```python
from build123d import *

# Parameters (mm, degrees)
SKETCH_1_R      = 3.4
EXTRUDE_1_DEPTH = 10


with BuildPart() as part:
    # 草图1 → 凸台-拉伸1 (new body)
    with BuildSketch(Plane.XY):
        with BuildLine():
            Line((-5.190537873, 20), (-27.590537873, 20))
            ThreePointArc((-27.590537873, 20), (-29.358304826, 19.267766953), (-30.090537873, 17.5))
            Line((-30.090537873, 17.5), (-30.090537873, 5.1))
            Line((-30.090537873, 5.1), (-29.090537873, 5.1))
            Line((-29.090537873, 5.1), (-29.090537873, 4.1))
            Line((-29.090537873, 4.1), (-25.890537873, 4.1))
            ThreePointArc((-25.890537873, 4.1), (-25.678405839, 4.187867966), (-25.590537873, 4.4))
            Line((-25.590537873, 4.4), (-25.590537873, 6.7))
            ThreePointArc((-25.590537873, 6.7), (-25.678405839, 6.912132034), (-25.890537873, 7))
            Line((-25.890537873, 7), (-27.290537873, 7))
            ThreePointArc((-27.290537873, 7), (-27.502669908, 7.087867966), (-27.590537873, 7.3))
            Line((-27.590537873, 7.3), (-27.590537873, 9.95))
            ThreePointArc((-27.590537873, 9.95), (-27.502669908, 10.162132034), (-27.290537873, 10.25))
            Line((-27.290537873, 10.25), (-22.856071779, 10.25))
            Line((-22.856071779, 10.25), (-17.840537873, 5.234466094))
            Line((-17.840537873, 5.234466094), (-17.840537873, 0))
            Line((-17.840537873, 0), (-17.840537873, -5.234466094))
            Line((-17.840537873, -5.234466094), (-22.856071779, -10.25))
            Line((-22.856071779, -10.25), (-27.290537873, -10.25))
            ThreePointArc((-27.290537873, -10.25), (-27.502669908, -10.162132034), (-27.590537873, -9.95))
            Line((-27.590537873, -9.95), (-27.590537873, -7.3))
            ThreePointArc((-27.590537873, -7.3), (-27.502669908, -7.087867966), (-27.290537873, -7))
            Line((-27.290537873, -7), (-25.890537873, -7))
            ThreePointArc((-25.890537873, -7), (-25.678405839, -6.912132034), (-25.590537873, -6.7))
            Line((-25.590537873, -6.7), (-25.590537873, -4.4))
            ThreePointArc((-25.590537873, -4.4), (-25.678405839, -4.187867966), (-25.890537873, -4.1))
            Line((-25.890537873, -4.1), (-29.090537873, -4.1))
            Line((-29.090537873, -4.1), (-29.090537873, -5.1))
            Line((-29.090537873, -5.1), (-30.090537873, -5.1))
            Line((-30.090537873, -5.1), (-30.090537873, -17.5))
            ThreePointArc((-30.090537873, -17.5), (-29.358304826, -19.267766953), (-27.590537873, -20))
            Line((-27.590537873, -20), (-5.190537873, -20))
            Line((-5.190537873, -20), (-5.190537873, -19))
            Line((-5.190537873, -19), (-4.190537873, -19))
            Line((-4.190537873, -19), (-4.190537873, -15.8))
            ThreePointArc((-4.190537873, -15.8), (-4.278405839, -15.587867966), (-4.490537873, -15.5))
            Line((-4.490537873, -15.5), (-6.790537873, -15.5))
            ThreePointArc((-6.790537873, -15.5), (-7.002669908, -15.587867966), (-7.090537873, -15.8))
            Line((-7.090537873, -15.8), (-7.090537873, -17.2))
            ThreePointArc((-7.090537873, -17.2), (-7.178405839, -17.412132034), (-7.390537873, -17.5))
            Line((-7.390537873, -17.5), (-10.040537873, -17.5))
            ThreePointArc((-10.040537873, -17.5), (-10.252669908, -17.412132034), (-10.340537873, -17.2))
            Line((-10.340537873, -17.2), (-10.340537873, -12.765533906))
            Line((-10.340537873, -12.765533906), (-5.325003967, -7.75))
            Line((-5.325003967, -7.75), (-0.090537873, -7.75))
            Line((-0.090537873, -7.75), (5.143928221, -7.75))
            Line((5.143928221, -7.75), (10.159462127, -12.765533906))
            Line((10.159462127, -12.765533906), (10.159462127, -17.2))
            ThreePointArc((10.159462127, -17.2), (10.071594161, -17.412132034), (9.859462127, -17.5))
            Line((9.859462127, -17.5), (7.209462127, -17.5))
            ThreePointArc((7.209462127, -17.5), (6.997330092, -17.412132034), (6.909462127, -17.2))
            Line((6.909462127, -17.2), (6.909462127, -15.8))
            ThreePointArc((6.909462127, -15.8), (6.821594161, -15.587867966), (6.609462127, -15.5))
            Line((6.609462127, -15.5), (4.309462127, -15.5))
            ThreePointArc((4.309462127, -15.5), (4.097330092, -15.587867966), (4.009462127, -15.8))
            Line((4.009462127, -15.8), (4.009462127, -19))
            Line((4.009462127, -19), (5.009462127, -19))
            Line((5.009462127, -19), (5.009462127, -20))
            Line((5.009462127, -20), (27.409462127, -20))
            ThreePointArc((27.409462127, -20), (29.17722908, -19.267766953), (29.909462127, -17.5))
            Line((29.909462127, -17.5), (29.909462127, -5.1))
            Line((29.909462127, -5.1), (28.909462127, -5.1))
            Line((28.909462127, -5.1), (28.909462127, -4.1))
            Line((28.909462127, -4.1), (25.709462127, -4.1))
            ThreePointArc((25.709462127, -4.1), (25.497330092, -4.187867966), (25.409462127, -4.4))
            Line((25.409462127, -4.4), (25.409462127, -6.7))
            ThreePointArc((25.409462127, -6.7), (25.497330092, -6.912132034), (25.709462127, -7))
            Line((25.709462127, -7), (27.109462127, -7))
            ThreePointArc((27.109462127, -7), (27.321594161, -7.087867966), (27.409462127, -7.3))
            Line((27.409462127, -7.3), (27.409462127, -9.95))
            ThreePointArc((27.409462127, -9.95), (27.321594161, -10.162132034), (27.109462127, -10.25))
            Line((27.109462127, -10.25), (22.674996033, -10.25))
            Line((22.674996033, -10.25), (17.659462127, -5.234466094))
            Line((17.659462127, -5.234466094), (17.659462127, 0))
            Line((17.659462127, 0), (17.659462127, 5.234466094))
            Line((17.659462127, 5.234466094), (22.674996033, 10.25))
            Line((22.674996033, 10.25), (27.109462127, 10.25))
            ThreePointArc((27.109462127, 10.25), (27.321594161, 10.162132034), (27.409462127, 9.95))
            Line((27.409462127, 9.95), (27.409462127, 7.3))
            ThreePointArc((27.409462127, 7.3), (27.321594161, 7.087867966), (27.109462127, 7))
            Line((27.109462127, 7), (25.709462127, 7))
            ThreePointArc((25.709462127, 7), (25.497330092, 6.912132034), (25.409462127, 6.7))
            Line((25.409462127, 6.7), (25.409462127, 4.4))
            ThreePointArc((25.409462127, 4.4), (25.497330092, 4.187867966), (25.709462127, 4.1))
            Line((25.709462127, 4.1), (28.909462127, 4.1))
            Line((28.909462127, 4.1), (28.909462127, 5.1))
            Line((28.909462127, 5.1), (29.909462127, 5.1))
            Line((29.909462127, 5.1), (29.909462127, 17.5))
            ThreePointArc((29.909462127, 17.5), (29.17722908, 19.267766953), (27.409462127, 20))
            Line((27.409462127, 20), (5.009462127, 20))
            Line((5.009462127, 20), (5.009462127, 19))
            Line((5.009462127, 19), (4.009462127, 19))
            Line((4.009462127, 19), (4.009462127, 15.8))
            ThreePointArc((4.009462127, 15.8), (4.097330092, 15.587867966), (4.309462127, 15.5))
            Line((4.309462127, 15.5), (6.609462127, 15.5))
            ThreePointArc((6.609462127, 15.5), (6.821594161, 15.587867966), (6.909462127, 15.8))
            Line((6.909462127, 15.8), (6.909462127, 17.2))
            ThreePointArc((6.909462127, 17.2), (6.997330092, 17.412132034), (7.209462127, 17.5))
            Line((7.209462127, 17.5), (9.859462127, 17.5))
            ThreePointArc((9.859462127, 17.5), (10.071594161, 17.412132034), (10.159462127, 17.2))
            Line((10.159462127, 17.2), (10.159462127, 12.765533906))
            Line((10.159462127, 12.765533906), (5.143928221, 7.75))
            Line((5.143928221, 7.75), (-0.090537873, 7.75))
            Line((-0.090537873, 7.75), (-5.325003967, 7.75))
            Line((-5.325003967, 7.75), (-10.340537873, 12.765533906))
            Line((-10.340537873, 12.765533906), (-10.340537873, 17.2))
            ThreePointArc((-10.340537873, 17.2), (-10.252669908, 17.412132034), (-10.040537873, 17.5))
            Line((-10.040537873, 17.5), (-7.390537873, 17.5))
            ThreePointArc((-7.390537873, 17.5), (-7.178405839, 17.412132034), (-7.090537873, 17.2))
            Line((-7.090537873, 17.2), (-7.090537873, 15.8))
            ThreePointArc((-7.090537873, 15.8), (-7.002669908, 15.587867966), (-6.790537873, 15.5))
            Line((-6.790537873, 15.5), (-4.490537873, 15.5))
            ThreePointArc((-4.490537873, 15.5), (-4.278405839, 15.587867966), (-4.190537873, 15.8))
            Line((-4.190537873, 15.8), (-4.190537873, 19))
            Line((-4.190537873, 19), (-5.190537873, 19))
            Line((-5.190537873, 19), (-5.190537873, 20))
        make_face()
        with Locations((-0.090537873, 0)):
            Circle(SKETCH_1_R, mode=Mode.SUBTRACT)
        Polygon((-12.840537873, 17.5), (-27.590537873, 17.5), (-27.590537873, 12.75), (-21.820537873, 12.75), (-18.550537873, 9.48), (-12.840537873, 9.48), (-12.840537873, 10.25), (-12.840537873, 12.75), align=None, mode=Mode.SUBTRACT)
        Polygon((-15.340537873, 6.98), (-15.340537873, 0), (-15.340537873, -6.98), (-10.340537873, -6.98), (-10.340537873, -4.48), (-5.990537873, -4.48), (-5.990537873, 0), (-5.990537873, 4.48), (-10.340537873, 4.48), (-10.340537873, 6.98), align=None, mode=Mode.SUBTRACT)
        Polygon((12.659462127, 17.5), (27.409462127, 17.5), (27.409462127, 12.75), (21.639462127, 12.75), (18.369462127, 9.48), (12.659462127, 9.48), (12.659462127, 10.25), (12.659462127, 12.75), align=None, mode=Mode.SUBTRACT)
        Polygon((15.159462127, 6.98), (15.159462127, 0), (15.159462127, -6.98), (10.159462127, -6.98), (10.159462127, -4.48), (5.809462127, -4.48), (5.809462127, 0), (5.809462127, 4.48), (10.159462127, 4.48), (10.159462127, 6.98), align=None, mode=Mode.SUBTRACT)
        Polygon((-12.840537873, -17.5), (-27.590537873, -17.5), (-27.590537873, -12.75), (-21.820537873, -12.75), (-18.550537873, -9.48), (-12.840537873, -9.48), (-12.840537873, -10.25), (-12.840537873, -12.75), align=None, mode=Mode.SUBTRACT)
        Polygon((12.659462127, -17.5), (27.409462127, -17.5), (27.409462127, -12.75), (21.639462127, -12.75), (18.369462127, -9.48), (12.659462127, -9.48), (12.659462127, -10.25), (12.659462127, -12.75), align=None, mode=Mode.SUBTRACT)
    extrude(amount=EXTRUDE_1_DEPTH)


solid = part.part
```
Geometry: final body of the model. Coordinates: model frame, mm. A direction names the side the tool comes from. Coordinates: 2 decimals unless noted, no trailing zeros. Order: outer loops, then holes, each group sorted by start corner. A loop starts at its lowest first (then second) coordinate and runs counter-clockwise, first axis right, second up. Notation, with made-up numbers: (13.25, 50.5) -> (43.25, 50.5) arc R4 ccw to (43.25, 56.5) -> close; hole circle Ø11 at (11.25, -23.75). An arc over 180 degrees is marked (long way). Answer in a Markdown table with one row per item.
Item 1: Section A-A on y = 0. Output: boundary loops of the cut face in (x, z), plus the area to 3 significant figures.
Return value:
| item | result |
|---|---|
| outline | (-17.84, 0) -> (-15.34, 0) -> (-15.34, 10) -> (-17.84, 10) -> close; (-5.99, 0) -> (-3.49, 0) -> (-3.49, 10) -> (-5.99, 10) -> close; (3.31, 0) -> (5.81, 0) -> (5.81, 10) -> (3.31, 10) -> close; (15.16, 0) -> (17.66, 0) -> (17.66, 10) -> (15.16, 10) -> close |
| area | 100 mm² |
Item 2: Ray query, L1, parallel to X at y = -14, z = 0.75; L2, parallel to Y at x = 4.5, z = 0.5; L3, parallel to Y at x = -23.5, z = 3.5. Return the intervals inside material, ascending.
Return value:
| item | result |
|---|---|
| L1 | x = -30.09 to -27.59, -12.84 to -10.34, 10.16 to 12.66, 27.41 to 29.91 |
| L2 | y = -19 to -15.5, -7.75 to 7.75, 15.5 to 19 |
| L3 | y = -20 to -17.5, -12.75 to -10.25, 10.25 to 12.75, 17.5 to 20 |
Item 3: Section C-C on x = -11. Output: boundary loops of the cut face in (y, z), plus the area to 3 significant figures.
Return value:
| item | result |
|---|---|
| outline | (-20, 0) -> (-6.98, 0) -> (-6.98, 10) -> (-20, 10) -> close; (6.98, 0) -> (20, 0) -> (20, 10) -> (6.98, 10) -> close |
| area | 260 mm² |
Item 4: Access query for faces 1 (the flat face through (2, -3, 0)), 2 (the flat face through (-16, -9.48, 5)). Directions: +Z, -Z, +X, -X, +Y, -Y. A direction counts if a zero-diameter tool reaches every point of the face in a straight line with its end or side. Return the directions, or none.
Return value:
| item | result |
|---|---|
| face 1 | -Z, +X, -X, +Y, -Y |
| face 2 | +Z, -Z |
Item 5: Contact query for flat-ended pins moving along their axis: P1, Ø3, axis at y = -1.5, z = 5, coming from the +X side; P2, Ø2, axis at x = 22.5, y = 7, coming from the -Z side; P3, Ø5, axis at y = 1.5, z = 2.5, coming from the -X side. Output: stop coordinate, or through.
Return value:
| item | result |
|---|---|
| P1 | stops at x = 17.66 |
| P2 | passes through |
| P3 | stops at x = -17.84 |
Item 6: Section D-D on z = 5.75. State how many separate pieces and enclosed holes the cut face has, plus the area to 3 significant figures.
Return value:
| item | result |
|---|---|
| separate pieces | 1 |
| enclosed holes | 7 |
| area | 1,020 mm² |
Item 7: Draft query along X for faces 3 (the flat face through (-25, -12.75, 5)), 4 (the flat face through (16, -20, 5)), 5 (the cylindrical face through (29.197, 19.248, 4.93)), 6 (the cylindrical face through (-29.378, -19.248, 4.93)). Return one class per face: released by +X, released by -X, zero draft, split by the parting line, or undercut.
Return value:
| item | result |
|---|---|
| face 3 | undercut |
| face 4 | zero draft |
| face 5 | released by +X |
| face 6 | released by -X |
Item 8: Section B-B on x = -24. Output: boundary loops of the cut face in (y, z).
Return value:
| item | result |
|---|---|
| outline | (-20, 0) -> (-17.5, 0) -> (-17.5, 10) -> (-20, 10) -> close; (-12.75, 0) -> (-10.25, 0) -> (-10.25, 10) -> (-12.75, 10) -> close; (10.25, 0) -> (12.75, 0) -> (12.75, 10) -> (10.25, 10) -> close; (17.5, 0) -> (20, 0) -> (20, 10) -> (17.5, 10) -> close |
